```python
from build123d import *

# Parameters (mm, degrees)
SKETCH1_R           = 15
BOSS_EXTRUDE1_DEPTH = 16
SKETCH2_R           = 13
CUT_EXTRUDE1_DEPTH  = 13.6
CHAMFER1_SIZE       = 1.5


with BuildPart() as part:
    # Sketch1 → Boss-Extrude1 (new body)
    with BuildSketch(Plane(origin=(0, 0, 0), x_dir=(1, 0, 0), z_dir=(0, 1, 0))):
        with Locations(Location((0, 0, 0), (0, 0, 270))):
            Circle(SKETCH1_R)
        with BuildLine():
            Line((-1.268857754, 0.8), (1.268857754, 0.8))
            ThreePointArc((1.268857754, 0.8), (0, -1.5), (-1.268857754, 0.8))
        make_face(mode=Mode.SUBTRACT)
    extrude(amount=BOSS_EXTRUDE1_DEPTH)

    # Sketch2 → Cut-Extrude1 (cut)
    with BuildSketch(Plane(origin=(0, 16, 0), x_dir=(1, 0, 0), z_dir=(0, 1, 0))):
        with Locations(Location((0, 0, 0), (0, 0, 270))):
            Circle(SKETCH2_R)
    extrude(amount=-CUT_EXTRUDE1_DEPTH, mode=Mode.SUBTRACT)

    # Chamfer1
    chamfer1_edges = [part.edges().sort_by_distance(p)[0] for p in [
        (0, 0, -15),
    ]]
    chamfer(chamfer1_edges, length=CHAMFER1_SIZE)


solid = part.part
```
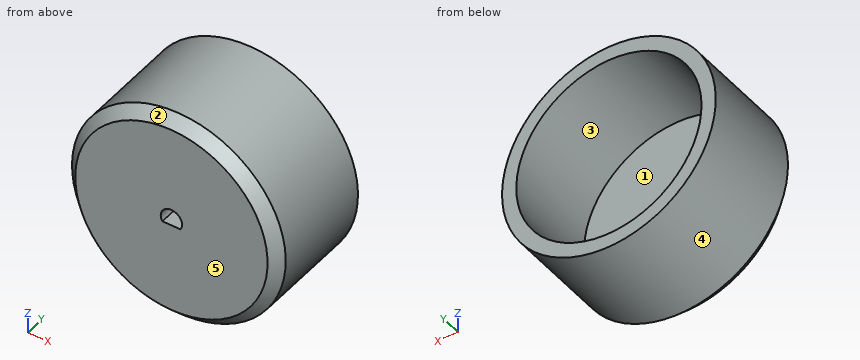
Can you work these out from the model? Positions are in its coordinate system, mm. Face numbers are marked on the shaded views. A direction names the side the tool comes from. Round coordinates to 2 decimals unless told otherwise and drop trailing zeros. Loops run counter-clockwise (first coordinate to the right, second up) from the corner with the lowest first, then second, coordinate; pieces in that order, holes last.
Item 1: Please list where these lines run through material, in increasing order: L1, parallel to X at y = 10.25, z = 0; L2, parallel to X at y = 4, z = -7; L3, parallel to Z at x = -10.75, y = 8.25.
Item 2: Which directions (+Z, -Z, +X, -X, +Y, -Y) give clear straight access to the entire face, cutting with the end or side of a thin tool? Please do the marked faces 1 and 2.
Item 3: Will these pins go through, and if not, where does the flat tip stop? pin 1 Ø8 at (x, y) = (-11.5, 3) entering from +Z; pin 2 Ø5 at (x, z) = (6, -2.5) entering from +Y; pin 3 Ø6 at (x, y) = (-2, 9.5) entering from +Z; pin 4 Ø0.7 at (x, y) = (0, 1) entering from +Z.
Item 4: Suppose I cut it at B-B, the plane x = 0. Write out the boundary of the cut face in (y, z), then the cut area to 3 significant figures.
Item 5: Suppose I cut it at D-D, the plane y = 2. Write out the boundary of the cut face in (x, z).
Item 6: If we mould it in two halves opening along X, with no side actions, what happens to the marked faces 3, 4 and 5? For each: +X half, -X half, draft (parallel to the pull), parting line (faces both ways), or undercut.
Item 7: Suppose I cut it at A-A, the plane z = 0. Write out the boundary of the cut face in (x, y).
Item 8: Suppose I cut it at C-C, the plane y = 9.75. Write out the boundary of the cut face in (x, z), then the cut area to 3 significant figures.
Reported:
1. L1: x = -15 to -13, 13 to 15
1. L2: x = -13.27 to -10.95, 10.95 to 13.27
1. L3: z = -10.46 to -7.31, 7.31 to 10.46
2. face 1: +Y
2. face 2: -Y
3. pin 1: stops at z = 12.99
3. pin 2: stops at y = 2.4
3. pin 3: stops at z = 15
3. pin 4: stops at z = 14.85
4. outline: (0, -13.5) - (1.5, -15) - (16, -15) - (16, -13) - (2.4, -13) - (2.4, -0.8) - (0, -0.8) - close; (0, 1.5) - (2.4, 1.5) - (2.4, 13) - (16, 13) - (16, 15) - (1.5, 15) - (0, 13.5) - close
4. area: 119 mm2
5. outline: circle Ø30 at (0, 0); hole (-1.27, -0.8) - (1.27, -0.8) arc R1.5 ccw (long way) to start
6. face 3: undercut
6. face 4: parting line
6. face 5: draft
7. outline: (-15, 1.5) - (-13.5, 0) - (-1.5, 0) - (-1.5, 2.4) - (-13, 2.4) - (-13, 16) - (-15, 16) - close; (1.5, 0) - (13.5, 0) - (15, 1.5) - (15, 16) - (13, 16) - (13, 2.4) - (1.5, 2.4) - close
8. outline: circle Ø30 at (0, 0); hole circle Ø26 at (0, 0)
8. area: 176 mm2
